```python
from build123d import *

# Parameters (mm, degrees)
BOSS_EXTRUDE1_DEPTH      = 50.8
BOSS_EXTRUDE1_DEPTH_BACK = 38.1
SKETCH2_W                = 381
SKETCH2_H                = 12.7
SKETCH3_W                = 12.7
SKETCH3_H                = 44.45
CUT_EXTRUDE1_DEPTH       = 2664.230012597
CAVITY1_START            = 115.8
CAVITY1_OUTLINE_R        = 12.7
CAVITY1_DEPTH            = 12.7
MOVE_FACE_HOLES_BY       = 0.635
MOVE_FACE_HOLES_2_BY     = 0.635
MOVE_FACE_SLOTS_BY       = 0.762
MOVE_FACE_SLOTS_2_BY     = 0.762
MOVE_FACE_SLOTS_3_BY     = 0.762
SLOT_FILLET_R            = 3.175


# Read off the part's stored shape, not the designer's step: Cavity1
with BuildPart() as part:
    # Sketch2 → Boss-Extrude1 (new, two sides: drawn at the far end of the back side and taken through both)
    with BuildSketch(Plane.XY.offset(287.7).offset(-BOSS_EXTRUDE1_DEPTH_BACK)):
        with Locations((2451.1, 122.15)):
            Rectangle(SKETCH2_W, SKETCH2_H)
    extrude(amount=BOSS_EXTRUDE1_DEPTH + BOSS_EXTRUDE1_DEPTH_BACK)

    # Sketch3 → Cut-Extrude1 (cut, through all)
    with BuildSketch(Plane(origin=(0, 128.5, 0), x_dir=(1, 0, 0), z_dir=(0, 1, 0))):
        with Locations((2470.15, -271.825)):
            Rectangle(SKETCH3_W, SKETCH3_H)
    extrude(amount=-CUT_EXTRUDE1_DEPTH, mode=Mode.SUBTRACT)

    # Cavity1 outline → Cavity1 (cut)
    with BuildSketch(Plane(origin=(0, 0, 0), x_dir=(1, 0, 0), z_dir=(0, 1, 0)).offset(CAVITY1_START)):
        with Locations((2300, -275)):
            Circle(CAVITY1_OUTLINE_R)
        with Locations((2600, -275)):
            Circle(CAVITY1_OUTLINE_R)
    extrude(amount=CAVITY1_DEPTH, mode=Mode.SUBTRACT)

    # Move Face Holes: a curved face moved inward by 0.635
    add(Solid.thicken(part.faces().sort_by_distance((2587.3, 122.15, 275))[0], -MOVE_FACE_HOLES_BY), mode=Mode.SUBTRACT)

    # Move Face Holes 2: a curved face moved inward by 0.635
    add(Solid.thicken(part.faces().sort_by_distance((2287.3, 122.15, 275))[0], -MOVE_FACE_HOLES_2_BY), mode=Mode.SUBTRACT)

    # Move Face Slots: a face moved inward by 0.762
    extrude(part.faces().sort_by_distance((2463.8, 122.15, 271.825))[0], amount=MOVE_FACE_SLOTS_BY, dir=(-1, 0, 0), mode=Mode.SUBTRACT)

    # Move Face Slots 2: a face moved inward by 0.762
    extrude(part.faces().sort_by_distance((2470.15, 122.15, 294.05))[0], amount=MOVE_FACE_SLOTS_2_BY, dir=(0, 0, 1), mode=Mode.SUBTRACT)

    # Move Face Slots 3: a face moved inward by 0.762
    extrude(part.faces().sort_by_distance((2476.5, 122.15, 271.825))[0], amount=MOVE_FACE_SLOTS_3_BY, dir=(1, 0, 0), mode=Mode.SUBTRACT)

    # Slot Fillet
    slot_fillet_edges = [part.edges().sort_by_distance(p)[0] for p in [
        (2477.262, 122.15, 294.812),
        (2463.038, 122.15, 294.812),
    ]]
    fillet(slot_fillet_edges, radius=SLOT_FILLET_R)


solid = part.part
```
CAD build for the part. Positions are in the model's coordinates, mm. A direction names the side the tool comes from. Round coordinates to 2 decimals unless told otherwise and drop trailing zeros. Order: outer loops, then holes, each group sorted by start corner. A loop starts at its lowest first (then second) coordinate and runs counter-clockwise, first axis right, second up. Notation, with made-up numbers: (-9.75, 51.25) -> (48.25, 51.25) arc R23 ccw to (48.25, 59.25) -> close; hole circle Ø9 at (-1, -8.5). An arc over 180 degrees is marked (long way). Write item = value, one per line.
(1) Cut at A-A (z = 275). Write the cut outline in (x, y) (3 decimals), plus the area to 3 significant figures.
Answers follow:
outline = (2260.6, 115.8) -> (2286.665, 115.8) -> (2286.665, 128.5) -> (2260.6, 128.5) -> close; (2313.335, 115.8) -> (2463.038, 115.8) -> (2463.038, 128.5) -> (2313.335, 128.5) -> close; (2477.262, 115.8) -> (2586.665, 115.8) -> (2586.665, 128.5) -> (2477.262, 128.5) -> close; (2613.335, 115.8) -> (2641.6, 115.8) -> (2641.6, 128.5) -> (2613.335, 128.5) -> close
area = 3,980 mm²
(2) 3-axis set-ups, long thin cutter, end or side, ignore diameter. For faces 1 (the flat face through (2470, 122, 294.812)), 2 (the flat face through (2260.6, 122, 293)): which of +Z, -Z, +X, -X, +Y, -Y reach the whole face in a straight line?
Answers follow:
face_1 = -Z, +Y, -Y
face_2 = +Z, -Z, -X, +Y, -Y
(3) Drill centre lines: L1, parallel to X at y = 120.5, z = 275 (3 decimals); L2, parallel to Z at x = 2600, y = 125.5 (3 decimals); L3, parallel to X at y = 122.5, z = 281. Where is each one in solid material? Low to high.
Answers follow:
L1 = 2260.6 to 2286.665, 2313.335 to 2463.038, 2477.262 to 2586.665, 2613.335 to 2641.6
L2 = 249.6 to 261.665, 288.335 to 338.5
L3 = 2260.6 to 2288.09, 2311.91 to 2463.04, 2477.26 to 2588.09, 2611.91 to 2641.6
(4) Pull direction X, two halves, no side cores. Call faces 3 (the cylindrical face through (2612.719, 122.061, 270.995)), 4 (the flat face through (2448, 122, 338.5)), 5 (the flat face through (2641.6, 122, 293)), 6 (the flat face through (2463.038, 122, 271)): +X half, -X half, draft (parallel to the pull), parting line (faces both ways), or undercut.
Answers follow:
face_3 = undercut
face_4 = draft
face_5 = +X half
face_6 = undercut
(5) Cut at C-C (x = 2300). Write the cut outline in (y, z) (3 decimals), plus the area to 3 significant figures.
Answers follow:
outline = (115.8, 249.6) -> (128.5, 249.6) -> (128.5, 261.665) -> (115.8, 261.665) -> close; (115.8, 288.335) -> (128.5, 288.335) -> (128.5, 338.5) -> (115.8, 338.5) -> close
area = 790 mm²
(6) Cut at D-D (z = 258). Write the cut outline in (x, y).
Answers follow:
outline = (2260.6, 115.8) -> (2463.04, 115.8) -> (2463.04, 128.5) -> (2260.6, 128.5) -> close; (2477.26, 115.8) -> (2641.6, 115.8) -> (2641.6, 128.5) -> (2477.26, 128.5) -> close
(7) Cut at B-B (y = 119). Write the cut outline in (x, z) (3 decimals).
Answers follow:
outline = (2260.6, 249.6) -> (2463.038, 249.6) -> (2463.038, 291.637) arc R3.175 cw to (2466.213, 294.812) -> (2474.087, 294.812) arc R3.175 cw to (2477.262, 291.637) -> (2477.262, 249.6) -> (2641.6, 249.6) -> (2641.6, 338.5) -> (2260.6, 338.5) -> close; hole circle Ø26.67 at (2300, 275); hole circle Ø26.67 at (2600, 275)
